Autodesk Inventor part; units mm, degrees
ref_plane "Work Plane2" through (11.866, 9.4714, 3.25) normal (0.9239, 0.3827, 0) x (-0.3827, 0.9239, 0)
ref_plane "YZ Plane" through (0, 0, 0) normal (1, 0, 0) x (0, 1, 0)
ref_plane "XZ Plane" through (0, 0, 0) normal (0, 1, 0) x (-1, 0, 0)
sketch "Sketch1" plane through (0, 0, 0) normal (0, 0, 1) x (1, 0, 0)
  arc A0 (11, 0) -> (-11, 0) centre (0, 0) ccw
  arc A1 (14.0712, 3.5) -> (-14.0712, 3.5) centre (0, 0) ccw
  line L0 (-11, 0) -> (-18.5, 0)
  line L1 (-18.5, 0) -> (-18.5, 3.5)
  line L2 (11, 0) -> (18.5, 0)
  line L3 (18.5, 0) -> (18.5, 3.5)
  line L4 (-18.5, 3.5) -> (-14.0712, 3.5)
  line L5 (18.5, 3.5) -> (14.0712, 3.5)
  dimension "d2" = 11
  dimension "d3" = 14.5
  dimension "d4" = 7.5
  dimension "d5" = 3.5
  dimension "d6" = 18.5
extrude "Extrusion1" add sketch "Sketch1" along normal blind 6.5
sketch "Sketch2" plane through (0, 0, 6.5) normal (0, 0, 1) x (1, 0, 0)
  line L0 (-18.5, 3.5) -> (-18.5, 0)
  line L1 (-18.5, 0) -> (-11, 0)
  arc A0 (11, 0) -> (-11, 0) centre (0, 0) ccw
  line L2 (11, 0) -> (18.5, 0)
  line L3 (18.5, 0) -> (18.5, 3.5)
  line L4 (18.5, 3.5) -> (14.0712, 3.5)
  arc A1 (14.0712, 3.5) -> (-14.0712, 3.5) centre (0, 0) ccw
  line L5 (3.5, 14.0712) -> (3.5, 16.0712)
  line L6 (3.5, 16.0712) -> (-3.5, 16.0712)
  line L7 (-3.5, 16.0712) -> (-3.5, 14.0712)
  arc A2 (14.0712, 3.5) -> (-14.0712, 3.5) centre (0, 0) ccw
  line L8 (-14.0712, 3.5) -> (-18.5, 3.5)
  line L9 (0, 0) -> (18.5, 0)
  line L10 (0, 0) -> (23.4857, 9.7281)
  dimension "d11" = 22.5
ref_plane "Work Plane2" through (11.866, 9.4714, 3.25) normal (0.9239, 0.3827, 0) x (-0.3827, 0.9239, 0)
ref_plane "Work Plane1" through (-11, 0, 3.25) normal (0.9239, 0.3827, 0) x (-0.3827, 0.9239, 0)
sketch "Sketch3" plane through (11.866, 9.4714, 3.25) normal (0.9239, 0.3827, 0) x (-0.3827, 0.9239, 0)
  line L0 (-4.2095, 3.25) -> (-11.2892, 3.25)
  line L1 (-6.3608, -3.25) -> (4.4089, -3.25)
  line L2 (-6.3608, 3.25) -> (4.4089, 3.25)
  line L3 (-6.3608, -3.25) -> (-6.3608, 3.25)
  line L4 (-11.2892, -3.25) -> (-8.0556, -3.25)
  line L5 (-8.0556, -3.25) -> (-8.0556, 3.25)
  line L6 (-11.2892, 3.25) -> (-8.0556, 3.25)
  line L7 (-11.2892, -3.25) -> (-11.2892, 3.25)
  line L8 (-8.0556, -3.25) -> (-6.3608, -3.25)
  line L9 (-6.3608, -3.25) -> (-6.3608, 3.25)
  line L10 (-8.0556, 3.25) -> (-6.3608, 3.25)
  line L11 (-8.0556, -3.25) -> (-8.0556, 3.25)
  line L12 (4.4089, -3.25) -> (4.4089, 3.25)
  point P0 (-4.2095, -3.25)
  point P1 (-4.2095, 0)
  point P2 (-4.2095, 3.25)
  dimension "d13" = 3.25
hole "Hole1" at (13.4769, 5.5823, 3.25) direction (-0.9239, -0.3827, 0) diameter 2 end through all
sketch "Sketch5" plane through (-18.5, 3.5, 0) normal (0, 1, 0) x (1, 0, 0)
  line L0 (4.4288, 0) -> (0, 0)
  line L1 (0, 0) -> (0, -6.5)
  line L2 (37, 0) -> (37, -6.5)
  line L3 (37, 0) -> (32.5712, 0)
  point P0 (18.5, 0)
  point P1 (2.5, -3.25)
  point P2 (34.5, -3.25)
  point P3 (0, -3.25)
  dimension "d31" = 2.5
  dimension "d32" = 2.5
  dimension "d33" = 3.25
  dimension "d34" = 3.25
hole "Hole3" at (-16, 3.5, 3.25) at (16, 3.5, 3.25) direction (0, -1, 0) diameter 1.567 end through all
properties part number "29 - Sheave Strap 1" material "Steel AISI 1020 107 HR"
Design review of the part built by this model. Coordinates are the model's own, in mm. A direction names the side the tool comes from. Round coordinates to 2 decimals unless told otherwise and drop trailing zeros. Order: outer loops, then holes, each group sorted by start corner. A loop starts at its lowest first (then second) coordinate and runs counter-clockwise, first axis right, second up.
1) Consider section A-A (x = -16). State the section outline as (y, z) points.
The answers:
outline: (0, 0) - (3.5, 0) - (3.5, 2.47) - (0, 2.47) - close; (0, 4.03) - (3.5, 4.03) - (3.5, 6.5) - (0, 6.5) - close
2) Machinability: for faces 4 (the flat face through (17, 3.5, 3)), 5 (the flat face through (-17, 3.5, 3)), 6 (the flat face through (15, 0, 3)), which of the approach directions +Z, -Z, +X, -X, +Y, -Y give a long, thin tool a straight path to every point of the face, cutting with its end or side? Answer none if there is none.
The answers:
face 4: +Z, -Z, +X, +Y
face 5: +Z, -Z, -X, +Y
face 6: +Z, -Z, +X, -X, -Y
3) Draft analysis for pull direction X (two halves, no side actions). For faces 1 (the flat face through (1, 12, 0)), 2 (the cylindrical face through (-0.269, 14.497, 3.204)), 3 (the cylindrical face through (-15.235, 1.726, 3.08)), state which applies: released by +X, released by -X, zero draft, split by the parting line, or undercut.
The answers:
face 1: zero draft
face 2: split by the parting line
face 3: undercut
4) Consider section D-D (y = 9.75). State the section outline as (x, z) points, plus the area to 3 significant figures.
The answers:
outline: (-10.73, 0) - (-5.09, 0) - (-5.09, 6.5) - (-10.73, 6.5) - close; (5.09, 0) - (10.73, 0) - (10.73, 6.5) - (5.09, 6.5) - close
area: 73.3 mm2
5) Consider section C-C (z = 5.25). State the section outline as (x, y) points.
The answers:
outline: (-18.5, 0) - (-11, 0) arc R11 cw to (11, 0) - (18.5, 0) - (18.5, 3.5) - (14.07, 3.5) arc R14.5 ccw to (-14.07, 3.5) - (-18.5, 3.5) - close
6) For L1, parallel to Z at x = 16, y = 0.85; L2, parallel to X at y = 1.6, z = 3.25; L3, parallel to X at y = 1.9, z = 3.25, list the stretches that pass through material, from the lowest coordinate up.
The answers:
L1: z = 0 to 2.47, 4.03 to 6.5
L2: x = -18.5 to -16.78, -15.22 to -10.88, 10.88 to 15.22, 16.78 to 18.5
L3: x = -18.5 to -16.78, -15.22 to -10.83, 10.83 to 15.22, 16.78 to 18.5
7) Clearance check with flat-ended pins moving along their axes: pin 1 Ø2 at (x, z) = (-16, 4) entering from +Y; pin 2 Ø1.5 at (x, y) = (-14.5, 7.5) entering from -Z. State where each tip first meets the part, or that it passes through.
The answers:
pin 1: stops at y = 3.5
pin 2: passes through
8) Consider section B-B (y = 1.5). State the section outline as (x, z) points, plus the area to 3 significant figures.
The answers:
outline: (-18.5, 0) - (-10.9, 0) - (-10.9, 6.5) - (-18.5, 6.5) - close; (10.9, 0) - (18.5, 0) - (18.5, 6.5) - (10.9, 6.5) - close; hole circle Ø1.57 at (-16, 3.25); hole circle Ø1.57 at (16, 3.25)
area: 95.0 mm2
